Could you check a few things on this model? Use its own coordinates, in mm. A direction names the side the tool comes from. Give positions to 0.01 mm unless a question says otherwise; leave off trailing zeros. Loops run counter-clockwise (first coordinate to the right, second up) from the corner with the lowest first, then second, coordinate; pieces in that order, holes last. Notation, with made-up numbers: (-17.75, 45) -> (14.25, 45) arc R27 ccw to (14.25, 80) -> close; hole circle Ø10 at (-36, 17). An arc over 180 degrees is marked (long way). Put each result on its own line as item: value.
```python
from build123d import *

# Parameters (mm, degrees)
F0_R     = 7.5
F1_DEPTH = 5
F2_R     = 2.95
F3_DEPTH = 2
F5_DEPTH = 6.5


with BuildPart() as f1:
    # F0 (on Front) → F1 (new body, symmetric)
    with BuildSketch(Plane.XZ):
        Circle(F0_R)
    extrude(amount=F1_DEPTH, both=True)

    # F2 (on face) → F3 (cut)
    with BuildSketch(Plane.XZ.offset(5)):
        Circle(F2_R)
    extrude(amount=-F3_DEPTH, mode=Mode.SUBTRACT)

    # F4 (on face) → F5 (cut)
    with BuildSketch(Plane(origin=(0, 5, 0), x_dir=(-1, 0, 0), z_dir=(0, 1, 0))):
        Polygon((1, 4.25), (-1, 4.25), (-1, 1), (-4.25, 1), (-4.25, -1), (-1, -1), (-1, -4.25), (1, -4.25), (1, -1), (4.25, -1), (4.25, 1), (1, 1), align=None)
    extrude(amount=-F5_DEPTH, mode=Mode.SUBTRACT)


solid = f1.part
```
1. If we section it at B-B (z = 0): List the corners of the cut face in (x, y) for me.
Recorded:
outline: (-7.5, -5) -> (-2.95, -5) -> (-2.95, -3) -> (2.95, -3) -> (2.95, -5) -> (7.5, -5) -> (7.5, 5) -> (4.25, 5) -> (4.25, -1.5) -> (-4.25, -1.5) -> (-4.25, 5) -> (-7.5, 5) -> close
2. I need wall thicknesses on line 1 (Z direction, x = 0, y = -3.7); line 2 (X direction, y = 0.25, z = 0.25); line 3 (Y direction, x = -3, z = 0.25). Which ranges of each line are inside material? Lowest first, please.
Recorded:
line 1: z = -7.5 to -2.95, 2.95 to 7.5
line 2: x = -7.5 to -4.25, 4.25 to 7.5
line 3: y = -5 to -1.5
3. I'm going to push flat-ended pins straight in: pin 1 (1 mm diameter, centred on y = 2.5, z = 4, fed in from +X); pin 2 (5 mm diameter, centred on x = 5.5, y = 0, fed in from -Z); pin 3 (6 mm diameter, centred on x = 0.5, y = 2.5, fed in from -Z); pin 4 (1 mm diameter, centred on x = -2.5, y = 1, fed in from -Z). Where does each tip first touch, or does it pass through?
Recorded:
pin 1: stops at x = 6.63
pin 2: stops at z = -6.87
pin 3: stops at z = -7.5
pin 4: stops at z = -7.23
4. If we section it at C-C (x = 0): List the corners of the cut face in (y, z) for me, then the cut area to 4 significant figures.
Recorded:
outline: (-5, -7.5) -> (5, -7.5) -> (5, -4.25) -> (-1.5, -4.25) -> (-1.5, 4.25) -> (5, 4.25) -> (5, 7.5) -> (-5, 7.5) -> (-5, 2.95) -> (-3, 2.95) -> (-3, -2.95) -> (-5, -2.95) -> close
area: 82.95 mm^2
5. For faces 4 (the face through (-2.947, -4.014, 0.13)), 5 (the face through (2, 5, -2)), 6 (the face through (-1, 2, 3)), which set-ups out of +Z, -Z, +X, -X, +Y, -Y let a thin tool reach every point of the face, with its end or its side?
Recorded:
face 4: -Y
face 5: +Z, -Z, +X, -X, +Y
face 6: +Y
6. Thinking about a two-plate mould opening in Z: for faces 1 (the face through (3.2, -5, 0.1)), 2 (the face through (-7.493, -0.07, 0.33)), 3 (the face through (-3, 2, -1)), which applies, pulls with the +Z half, pulls with the -Z half, needs draft (parallel to the pull), parting line crosses it, or undercut?
Recorded:
face 1: needs draft
face 2: parting line crosses it
face 3: undercut
7. If we section it at D-D (y = -2): List the corners of the cut face in (x, z) for me.
Recorded:
outline: circle Ø15 at (0, 0)
8. If we section it at A-A (y = 4): List the corners of the cut face in (x, z) for me.
Recorded:
outline: circle Ø15 at (0, 0); hole (-4.25, -1) -> (-1, -1) -> (-1, -4.25) -> (1, -4.25) -> (1, -1) -> (4.25, -1) -> (4.25, 1) -> (1, 1) -> (1, 4.25) -> (-1, 4.25) -> (-1, 1) -> (-4.25, 1) -> close
